Read the model definition and answer for the solid it produces. Units are mm, in the model's axes. Face numbers are marked on the shaded views. A direction names the side the tool comes from. Coordinates: 2 decimals unless noted, no trailing zeros. Loops run counter-clockwise (first coordinate to the right, second up) from the corner with the lowest first, then second, coordinate; pieces in that order, holes last. Notation, with made-up numbers: (20, 66.25) -> (50, 66.25) arc R22 ccw to (50, 81.25) -> close; hole circle Ø5 at (-31, 38). An arc over 180 degrees is marked (long way). Answer as a JSON object with one key per item and string values. Group by question number.
Q1. This flat-tipped pin is pushed along its axis until it touches: P1, Ø1.8, axis at x = 7, y = 49.5, coming from the +Z side. Where does it stop, or does it pass through?
Q2. The part is cut by section B-B on x = 0. Write down the section's boundary in (y, z) (3 decimals), and give its area (3 significant figures).
Q3. The part is cut by section A-A on x = 37. Write down the section's boundary in (y, z), and give its area (3 significant figures).
Q4. The part is cut by section D-D on z = -29. Write down the section's boundary in (x, y).
Q5. Determine the mould class of the marked faces 1, 2, 3 and 4 for opening direction X: released by +X, released by -X, zero draft, split by the parting line, or undercut.
Q6. Straight lines are drawn through the part: line 1 along X through (y, z) = (-7, 25.5); line 2 along Z through (x, y) = (0, 48) (3 decimals); line 3 along Y through (x, z) = (17.5, -16). For each, find the intervals that lie inside material, in ascending order. Write a range as [from, to].
Q7. For the marked faces 5 and 6, determine the directions among +Z, -Z, +X, -X, +Y, -Y from which every point of the face is accessible in a straight line to the end or side of a thin tool.
Q8. The part is cut by section C-C on y = -18. Write down the section's boundary in (x, z), and give its area (3 significant figures).
from build123d import *

# Parameters (mm, degrees)
F1_DEPTH = 50.8
F2_W     = 93.022012
F2_H     = 94.683118
F3_DEPTH = 114.3
F4_R     = 8.12477
F5_DEPTH = 228.6
F6_R     = 8.143617
F7_DEPTH = 152.4


with BuildPart() as f1:
    # F0 (on Front) → F1 (new body, symmetric)
    with BuildSketch(Plane.XZ):
        Polygon((23.393929, 13.422799), (-19.51801, 13.422799), (-19.51801, 33.632938), (-49.14109, 33.632938), (-49.14109, 13.422799), (-49.14109, -37.794676), (53.017005, -37.794676), (53.017005, 13.422799), (53.017005, 33.632938), (23.393929, 33.632938), align=None)
    extrude(amount=F1_DEPTH, both=True)

    # F2 (on Top) → F3 (cut, symmetric)
    with BuildSketch(Plane.XY):
        with Locations((2.353236, -0.14291)):
            Rectangle(F2_W, F2_H)
    extrude(amount=F3_DEPTH, both=True, mode=Mode.SUBTRACT)

    # F4 (on Front) → F5 (cut)
    with BuildSketch(Plane.XZ):
        with Locations((0, -15.092876)):
            Circle(F4_R)
    extrude(amount=-F5_DEPTH, mode=Mode.SUBTRACT)

    # F6 (on face) → F7 (cut)
    with BuildSketch(Plane.XZ.offset(50.8)):
        with Locations((0, -13.708619)):
            Circle(F6_R)
    extrude(amount=-F7_DEPTH, mode=Mode.SUBTRACT)


solid = f1.part
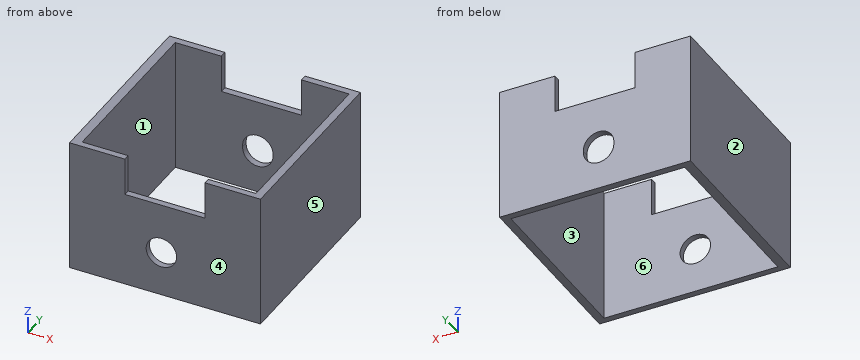
Final values:
{
 "1": {"P1": "stops at z = 13.42"},
 "2": {"outline": "(-50.8, -37.795) -> (-47.484, -37.795) -> (-47.484, -21.852) -> (-50.8, -21.852) -> close; (-50.8, -5.565) -> (-47.484, -5.565) -> (-47.484, 13.423) -> (-50.8, 13.423) -> close; (47.199, -37.795) -> (50.8, -37.795) -> (50.8, -23.218) -> (47.199, -23.218) -> close; (47.199, -5.565) -> (50.8, -5.565) -> (50.8, 13.423) -> (47.199, 13.423) -> close", "area": "237 mm2"},
 "3": {"outline": "(-50.8, -37.79) -> (-47.48, -37.79) -> (-47.48, 33.63) -> (-50.8, 33.63) -> close; (47.2, -37.79) -> (50.8, -37.79) -> (50.8, 33.63) -> (47.2, 33.63) -> close", "area": "494 mm2"},
 "4": {"outline": "(-49.14, -50.8) -> (53.02, -50.8) -> (53.02, 50.8) -> (-49.14, 50.8) -> close; hole (-44.16, -47.48) -> (48.86, -47.48) -> (48.86, 47.2) -> (-44.16, 47.2) -> close"},
 "5": {"face 1": "undercut", "face 2": "released by -X", "face 3": "undercut", "face 4": "zero draft"},
 "6": {"line 1": "x = [-49.14, -44.16], [48.86, 53.02]", "line 2": "z = [-37.795, -23.218], [-5.565, 13.423]", "line 3": "y = [-50.8, -47.48], [47.2, 50.8]"},
 "7": {"face 5": "+Z, -Z, +X, +Y, -Y", "face 6": "+Z, -Z"},
 "8": {"outline": "(-49.14, -37.79) -> (-44.16, -37.79) -> (-44.16, 33.63) -> (-49.14, 33.63) -> close; (48.86, -37.79) -> (53.02, -37.79) -> (53.02, 33.63) -> (48.86, 33.63) -> close", "area": "653 mm2"}
}
